Geometry: final body of the model. Coordinates: model frame, mm. A direction names the side the tool comes from. Round coordinates to 2 decimals unless told otherwise and drop trailing zeros. Order: outer loops, then holes, each group sorted by start corner. A loop starts at its lowest first (then second) coordinate and runs counter-clockwise, first axis right, second up. Notation, with made-up numbers: M 15,-3.75 L 19,-3.75 A11 cw 19,8.25 Z; hole C -14,16.5 d4. An arc over 180 degrees is marked long. Return JSON: item names as keys, results as strings. Group by question number.
Q1. Access query for faces 1 (the face through (-93, -65, -8)), 2 (the face through (-10, 0, 5)), 3 (the face through (-92, 61.57, -8)). Directions: +Z, -Z, +X, -X, +Y, -Y. A direction counts if a zero-diameter tool reaches every point of the face in a straight line with its end or side. Return the directions, or none.
Q2. Contact query for flat-ended pins moving along their axis: pin 1 (8 mm diameter, centred on y = 2.5, z = -11.5, fed in from +X); pin 2 (5 mm diameter, centred on x = -27, y = 32, fed in from -Z); pin 3 (3.5 mm diameter, centred on x = 73, y = 90, fed in from +Z); pin 4 (1 mm diameter, centred on x = 0.5, z = 5.5, fed in from +Y). Output: stop coordinate, or through.
Q3. Cut plane A-A on z = -8. Output: boundary loops of the cut face in (x, y), and give its area (3 significant figures).
Q4. Cut plane C-C on y = 12. Output: boundary loops of the cut face in (x, z).
Q5. Mould query, pull axis X, two halves, no side actions, for faces 4 (the face through (-26, -1, 6)), 5 (the face through (-102, -1, -8)), 6 (the face through (102, -4, 2)). Classes: released by +X, released by -X, zero draft, split by the parting line, or undercut.
Q6. Cut plane D-D on y = -44.5. Output: boundary loops of the cut face in (x, z).
Q7. Cut plane B-B on x = -79. Output: boundary loops of the cut face in (y, z), and give its area (3 significant figures).
Q8. Ray query, probe 1 along Y at (x, z) = (73, 0.55); probe 2 along X at (y, z) = (0, 1.1); probe 3 along X at (y, z) = (-53, -10). Return the intervals inside material, ascending.
Solid Edge part; units mm, degrees
sketch "Sketch1" plane through (0, 0, 0) normal (0, 0, 1) x (1, 0, 0)
  line L0 (-102, -125) -> (102, -125)
  line L1 (102, -125) -> (102, 125)
  line L2 (102, 125) -> (-102, 125)
  line L3 (-102, 125) -> (-102, -125)
  dimension "D1" = 102
  dimension "D2" = 102
extrude "Protrusion1" add sketch "Sketch1" along normal blind 3
sketch "Sketch2" plane through (0, 0, 3) normal (0, 0, 1) x (1, 0, 0)
  circle A0 centre (73, 90) radius 2.25
  circle A1 centre (73, -90) radius 2.25
  circle A2 centre (-41, -90) radius 2.25
  circle A3 centre (-41, 90) radius 2.25
  dimension "D1" = 41
  dimension "D2" = 41
extrude "Cutout1" cut sketch "Sketch2" against normal through all
sketch "Sketch3" plane through (0, 0, 3) normal (0, 0, 1) x (1, 0, 0)
  line L0 (-102, -65) -> (102, -65)
  line L1 (102, -65) -> (102, 61.57)
  line L2 (102, 61.57) -> (-102, 61.57)
  line L3 (-102, 61.57) -> (-102, -65)
extrude "Extrusionsausprägung_2" add sketch "Sketch3" along normal blind 3
sketch "Sketch4" plane through (0, 93.285, 3) normal (0, 0, 1) x (-1, 0, 0)
  line L0 (-102, -31.715) -> (102, -31.715)
  line L1 (102, -31.715) -> (102, -27.715)
  line L2 (102, -27.715) -> (-102, -27.715)
  line L3 (-102, -27.715) -> (-102, -31.715)
  dimension "D1" = 102
extrude "Cutout2" cut sketch "Sketch4" against normal through all
sketch "Sketch5" plane through (0, -1.715, 6) normal (0, 0, 1) x (-1, 0, 0)
  line L0 (5, -22.715) -> (5, 37.285)
  line L1 (5, 37.285) -> (-5, 37.285)
  line L2 (-5, 37.285) -> (-5, -22.715)
  line L3 (-5, -22.715) -> (-15, -22.715)
  line L4 (-15, -22.715) -> (0, -42.715)
  line L5 (0, -42.715) -> (15, -22.715)
  line L6 (15, -22.715) -> (5, -22.715)
  dimension "D1" = 5
  dimension "D2" = 5
  dimension "D3" = 15
extrude "Cutout3" cut sketch "Sketch5" against normal blind 2
sketch "Sketch6" plane through (0, -1.715, 6) normal (0, 0, 1) x (-1, 0, 0)
  circle A0 centre (4, -1.715) radius 2.25
  circle A1 centre (-36, -1.715) radius 2.25
extrude "Cutout4" cut sketch "Sketch6" against normal through all
sketch "Sketch7" plane through (0, -1.715, 6) normal (0, 0, 1) x (-1, 0, 0)
  circle A0 centre (4, -1.715) radius 6
extrude "Cutout5" cut sketch "Sketch7" against normal up to vertex (2 mm away)
chamfer "Fase_2" distance 0.5 angle 60 6 edges at (70.75, -90, 3) (-43.25, -90, 3) (38.25, 0, 6) (-1.75, 0, 4) (-43.25, 90, 3) (70.75, 90, 3) measured on face at (-70.04, -42.6393, 6)
sketch "Sketch8" plane through (0, -1.715, 6) normal (0, 0, 1) x (-1, 0, 0)
  line L0 (102, 63.285) -> (105, 63.285)
  line L1 (105, 63.285) -> (105, -63.285)
  line L2 (105, -63.285) -> (102, -63.285)
  line L3 (102, -63.285) -> (102, 63.285)
  dimension "D1" = 102
extrude "Extrusionsausprägung_3" add sketch "Sketch8" against normal blind 23
sketch "Sketch9" plane through (0, -2, 0) normal (0, 0, -1) x (1, 0, 0)
  line L0 (-95, 63) -> (-90, 63)
  line L1 (-90, 63) -> (-90, -63.57)
  line L2 (-90, -63.57) -> (-95, -63.57)
  line L3 (-95, -63.57) -> (-95, 63)
  dimension "D1" = 95
extrude "Protrusion2" add sketch "Sketch9" along normal up to vertex (17 mm away)
properties material "Nylon, allgemein"
Result sheet:
{
 "1": {"face 1": "-Z, +X, -X, -Y", "face 2": "+Z", "face 3": "-Z, +X, -X, +Y"},
 "2": {"pin 1": "stops at x = -90", "pin 2": "stops at z = 0", "pin 3": "passes through", "pin 4": "stops at y = 61.57"},
 "3": {"outline": "M -105,-65 L -102,-65 L -102,61.57 L -105,61.57 Z; M -95,-65 L -90,-65 L -90,61.57 L -95,61.57 Z", "area": "1,010 mm²"},
 "4": {"outline": "M -105,-17 L -102,-17 L -102,0 L -95,0 L -95,-17 L -90,-17 L -90,0 L 102,0 L 102,6 L 5,6 L 5,4 L -5,4 L -5,6 L -105,6 Z"},
 "5": {"face 4": "zero draft", "face 5": "undercut", "face 6": "released by +X"},
 "6": {"outline": "M -105,-17 L -102,-17 L -102,0 L -95,0 L -95,-17 L -90,-17 L -90,0 L 102,0 L 102,6 L -105,6 Z"},
 "7": {"outline": "M -125,0 L 121,0 L 121,3 L 61.57,3 L 61.57,6 L -65,6 L -65,3 L -125,3 Z", "area": "1,120 mm²"},
 "8": {"probe 1": "y = -125 to -92.25, -87.75 to 87.75, 92.25 to 121", "probe 2": "x = -105 to -6.25, -1.75 to 33.75, 38.25 to 102", "probe 3": "x = -105 to -102, -95 to -90"}
}
